The model under review builds one solid part; all positions refer to its coordinate system, in mm. A direction names the side the tool comes from. Give positions to 0.01 mm unless a question says otherwise; leave off trailing zeros. Loops run counter-clockwise (first coordinate to the right, second up) from the corner with the lowest first, then second, coordinate; pieces in that order, holes last. Notation, with made-up numbers: M -30,66 L -2,66 A37 ccw -2,102 Z; hole C 57,-31.75 d5. An arc over 180 degrees is marked long. Return JSON: item names as keys, results as strings. Group by question number.
```python
from build123d import *

# Parameters (mm, degrees)
SKETCH1_R               = 7.5
SKETCH1_R_2             = 5
BOSS_EXTRUDE1_DEPTH     = 80
BOSS_EXTRUDE2_DEPTH     = 160
CUT_EXTRUDE1_DEPTH      = 212.272992998
CUT_EXTRUDE1_DEPTH_BACK = 212.272992998


with BuildPart() as part:
    # Sketch1 → Boss-Extrude1 (new, symmetric)
    with BuildSketch(Plane(origin=(0, 0, 0), x_dir=(1, 0, 0), z_dir=(0, 1, 0))):
        with Locations(Location((130.052474297, -2.753634589, 0), (0, 0, 270))):
            Circle(SKETCH1_R)
        with Locations(Location((130.052474297, -2.753634589, 0), (0, 0, 270))):
            Circle(SKETCH1_R_2, mode=Mode.SUBTRACT)
    extrude(amount=BOSS_EXTRUDE1_DEPTH, both=True)

    # Sketch2 → Boss-Extrude2 (add)
    with BuildSketch(Plane(origin=(0, 80, 0), x_dir=(1, 0, 0), z_dir=(0, 1, 0))):
        Polygon((130.052474297, 4.746365411), (195.141045325, 5.361337723), (195.141045325, 2.246365411), (130.052474297, 2.246365411), align=None)
    extrude(amount=-BOSS_EXTRUDE2_DEPTH)

    # Sketch3 → Cut-Extrude1 (cut, two sides: drawn at the far end of the back side and taken through both)
    with BuildSketch(Plane.XY.offset(-2.246365411).offset(-CUT_EXTRUDE1_DEPTH_BACK)):
        Polygon((101.023989242, 40), (137.552474297, 40), (137.552474297, 0), (107.599116552, 0), (107.599116552, -40), (137.552474297, -40), (137.552474297, -90), (101.023989242, -90), align=None)
    extrude(amount=CUT_EXTRUDE1_DEPTH + CUT_EXTRUDE1_DEPTH_BACK, mode=Mode.SUBTRACT)


solid = part.part
```
(1) For pin 1 (7.5 mm diameter, centred on x = 128.5, z = -0.5, fed in from -Y); pin 2 (6 mm diameter, centred on x = 175, y = 53.5, fed in from -Z); pin 3 (3 mm diameter, centred on y = -4, z = -0.5, fed in from -X), all flat-tipped, find the tip position at first contact; note any pin that passes through.
(2) Add section C-C (x = 182). Write out the cut boundary in (y, z), and give its area (3 significant figures).
(3) Add section D-D (y = -50.5). Write out the cut boundary in (x, z), and give its area (3 significant figures).
(4) For probe 1 along Y at (x, z) = (132.5, 8.75); probe 2 along X at (y, z) = (-12, 2.25); probe 3 along Z at (x, y) = (139.5, 47), list the stretches that pass through material, from the lowest coordinate up.
(5) For faces 1 (the flat face through (135, -40, 1)), 2 (the flat face through (130.2, 0, -2.4)), 3 (the cylindrical face through (125.17, 59.72, 1.67)), list the 3-axis set-ups (+Z, -Z, +X, -X, +Y, -Y) from which the entire face can be reached by the end or side of a thin tool; tool diameter is ignored.
(6) Add section A-A (z = 4.25). Write out the cut boundary in (x, y), and give its area (3 significant figures).
(7) Add section B-B (y = 54). Write out the cut boundary in (x, z).
(8) Mouldability with a two-part tool opening along Y and no side actions: class faces 4 (the cylindrical face through (125.17, -20.28, 1.67)), 5 (the flat face through (154, 80, -3)), 6 (the flat face through (135, 40, 1)) as released by +Y, released by -Y, zero draft, split by the parting line, or undercut.
Verdict:
{
 "1": {"pin 1": "stops at y = -40", "pin 2": "stops at z = -5.2", "pin 3": "stops at x = 122.76"},
 "2": {"outline": "M -80,-5.24 L 80,-5.24 L 80,-2.25 L -80,-2.25 Z", "area": "479 mm²"},
 "3": {"outline": "M 137.55,-4.82 L 195.14,-5.36 L 195.14,-2.25 L 137.55,-2.25 Z", "area": "164 mm²"},
 "4": {"probe 1": "y = -40 to 0, 40 to 80", "probe 2": "x = 122.57 to 125.08, 135.03 to 137.54", "probe 3": "z = -4.84 to -2.25"},
 "5": {"face 1": "+Z, -Z, -X, -Y", "face 2": "+Z, -Z, -X", "face 3": "+Y, -Y"},
 "6": {"outline": "M 122.7,-40 L 125.28,-40 L 125.28,0 L 122.7,0 Z; M 122.7,40 L 125.28,40 L 125.28,80 L 122.7,80 Z; M 134.82,-40 L 137.4,-40 L 137.4,0 L 134.82,0 Z; M 134.82,40 L 137.4,40 L 137.4,80 L 134.82,80 Z", "area": "413 mm²"},
 "7": {"outline": "M 130.05,-4.75 L 195.14,-5.36 L 195.14,-2.25 L 135.64,-2.25 A7.5 ccw long Z; hole C 130.05,2.75 d10"},
 "8": {"face 4": "zero draft", "face 5": "released by +Y", "face 6": "undercut"}
}
